Work out the finished part from the listing and answer in its coordinate system (mm). A direction names the side the tool comes from. Give positions to 0.01 mm unless a question says otherwise; leave off trailing zeros. Write each loop counter-clockwise with the first axis right and the second up, starting at its lowest first coordinate (ties: lowest second). Pieces come first, ordered by that corner, then holes. Notation, with made-up numbers: (-35.75, -18) -> (-14.75, -18) arc R29 ccw to (-14.75, 5) -> close; hole circle Ø1 at (20, 30.5). An arc over 180 degrees is marked (long way). Use a Markdown table: item, result. Add a question column.
Q1. Section D-D, the plane y = 11 is taken. Give the vertices of the cut face in (x, z), plus the area to 3 significant figures.
Q2. Section A-A, the plane y = 0 is taken. Give the vertices of the cut face in (x, z), plus the area to 3 significant figures.
Q3. For faces 4 (the face through (-4, 4, -2.5)), 5 (the face through (-18, -3, 3)), 6 (the face through (-4, 4, 2.5)), 7 (the face through (-4.336, -19.524, -3.986)), 8 (the face through (3, 15, 5)), determine the directions among +Z, -Z, +X, -X, +Y, -Y from which every point of the face is accessible in a straight line to the end or side of a thin tool.
Q4. Consider line 1 (Z direction, x = -12, y = -14); line 2 (Y direction, x = 0, z = 1.4); line 3 (X direction, y = -0.5, z = 4.25). Determine where each line is inside the solid, lowest interval first.
Q5. For a pull along X with two mould halves and no side action, classify faces 1 (the face through (-4.336, -19.524, 4.014)), 2 (the face through (3, 15, -5)), 3 (the face through (-1.08, -4.88, 0.04)) as pulls with the +X half, pulls with the -X half, needs draft (parallel to the pull), parting line crosses it, or undercut.
Q6. Each of these flat-tipped pins is pushed along its axis until it touches: pin 1 Ø1.5 at (x, y) = (5.5, -10.5) entering from +Z; pin 2 Ø6 at (x, z) = (6.5, -2.5) entering from -Y; pin 3 Ø6 at (y, z) = (-9.5, 3) entering from -X. Where does it stop, or does it pass through?
Q7. Section C-C, the plane z = -4 is taken. Give the vertices of the cut face in (x, y).
from build123d import *

# Parameters (mm, degrees)
SKETCH_1_R          = 20
SKETCH_1_R_2        = 15
SKETCH_1_R_3        = 5
EXTRUDE_2_DEPTH     = 5
SKETCH_2_R          = 15
CUT_EXTRUDE_1_DEPTH = 5
SKETCH_3_R          = 15
CUT_EXTRUDE_6_DEPTH = 31
SKETCH_4_R          = 15
EXTRUDE_3_DEPTH     = 2.5
SKETCH_5_R          = 5
CUT_EXTRUDE_7_DEPTH = 30.261749777
SKETCH_8_W          = 2
SKETCH_8_H          = 6


with BuildPart() as part:
    # 草图1 → 凸台-拉伸2 (new, symmetric)
    # profile 1 of 2: a face of its own
    with BuildSketch(Plane.XY):
        Circle(SKETCH_1_R)
        Circle(SKETCH_1_R_2, mode=Mode.SUBTRACT)
    # profile 2 of 2: a face of its own
    with BuildSketch(Plane.XY):
        Circle(SKETCH_1_R_2)
        Circle(SKETCH_1_R_3, mode=Mode.SUBTRACT)
    extrude(amount=EXTRUDE_2_DEPTH, both=True)

    # 草图2 → 切除-拉伸1 (cut)
    with BuildSketch(Plane.XY.offset(5)):
        Circle(SKETCH_2_R)
    extrude(amount=-CUT_EXTRUDE_1_DEPTH, mode=Mode.SUBTRACT)

    # 草图3 → 切除-拉伸6 (cut, through all)
    with BuildSketch(Plane(origin=(0, 0, -5), x_dir=(-1, 0, 0), z_dir=(0, 0, -1))):
        with Locations(Location((0, 0, 0), (0, 0, 180))):
            Circle(SKETCH_3_R)
    extrude(amount=-CUT_EXTRUDE_6_DEPTH, mode=Mode.SUBTRACT)

    # 草图4 → 凸台-拉伸3 (add, symmetric)
    with BuildSketch(Plane.XY):
        Circle(SKETCH_4_R)
    extrude(amount=EXTRUDE_3_DEPTH, both=True)

    # 草图5 → 切除-拉伸7 (cut, through all)
    with BuildSketch(Plane.XY.offset(2.5)):
        Circle(SKETCH_5_R)
    extrude(amount=-CUT_EXTRUDE_7_DEPTH, mode=Mode.SUBTRACT)

    # 草图8 → 切除-旋转1 (revolve, cut)
    with BuildSketch(Plane(origin=(0, 0, 0), x_dir=(1, 0, 0), z_dir=(0, 1, 0)), mode=Mode.PRIVATE) as cut_revolve_1_sk:
        with Locations((-19, 0)):
            Rectangle(SKETCH_8_W, SKETCH_8_H)
    revolve(cut_revolve_1_sk.sketch.rotate(Axis((0, 0, 0), (0, 0, -1)), 180), axis=Axis((0, 0, 0), (0, 0, -1)), mode=Mode.SUBTRACT)


solid = part.part
Result set:
| question | item | result |
|---|---|---|
| 1 | outline | (-16.7, -5) -> (-10.2, -5) -> (-10.2, -2.5) -> (10.2, -2.5) -> (10.2, -5) -> (16.7, -5) -> (16.7, -3) -> (14.25, -3) -> (14.25, 3) -> (16.7, 3) -> (16.7, 5) -> (10.2, 5) -> (10.2, 2.5) -> (-10.2, 2.5) -> (-10.2, 5) -> (-16.7, 5) -> (-16.7, 3) -> (-14.25, 3) -> (-14.25, -3) -> (-16.7, -3) -> close |
| 1 | area | 203 mm2 |
| 2 | outline | (-20, -5) -> (-15, -5) -> (-15, -2.5) -> (-5, -2.5) -> (-5, 2.5) -> (-15, 2.5) -> (-15, 5) -> (-20, 5) -> (-20, 3) -> (-18, 3) -> (-18, -3) -> (-20, -3) -> close; (5, -2.5) -> (15, -2.5) -> (15, -5) -> (20, -5) -> (20, -3) -> (18, -3) -> (18, 3) -> (20, 3) -> (20, 5) -> (15, 5) -> (15, 2.5) -> (5, 2.5) -> close |
| 2 | area | 176 mm2 |
| 3 | face 4 | -Z |
| 3 | face 5 | none |
| 3 | face 6 | +Z |
| 3 | face 7 | +Z, -Z |
| 3 | face 8 | +Z, +X, -X, +Y, -Y |
| 4 | line 1 | z = -5 to -3, 3 to 5 |
| 4 | line 2 | y = -18 to -5, 5 to 18 |
| 4 | line 3 | x = -19.99 to -14.99, 14.99 to 19.99 |
| 5 | face 1 | parting line crosses it |
| 5 | face 2 | needs draft |
| 5 | face 3 | undercut |
| 6 | pin 1 | stops at z = 2.5 |
| 6 | pin 2 | stops at y = -19.68 |
| 6 | pin 3 | stops at x = -18.91 |
| 7 | outline | circle Ø40 at (0, 0); hole circle Ø30 at (0, 0) |
